Check sheet for the drawn part. Datum: minimum x, y, z corner. Units: mm. Coordinates: 2 decimals unless noted, no trailing zeros. Write each loop counter-clockwise with the first axis right and the second up, starting at its lowest first coordinate (ties: lowest second). Pieces come first, ordered by that corner, then holes. Notation, with made-up numbers: (7.25, -8.5) - (34.25, -8.5) arc R27 ccw to (34.25, 21.5) - close; hole circle Ø10 at (-6, 5.25). An arc over 180 degrees is marked (long way). Write each question's results on one line, items separated by ' | '.
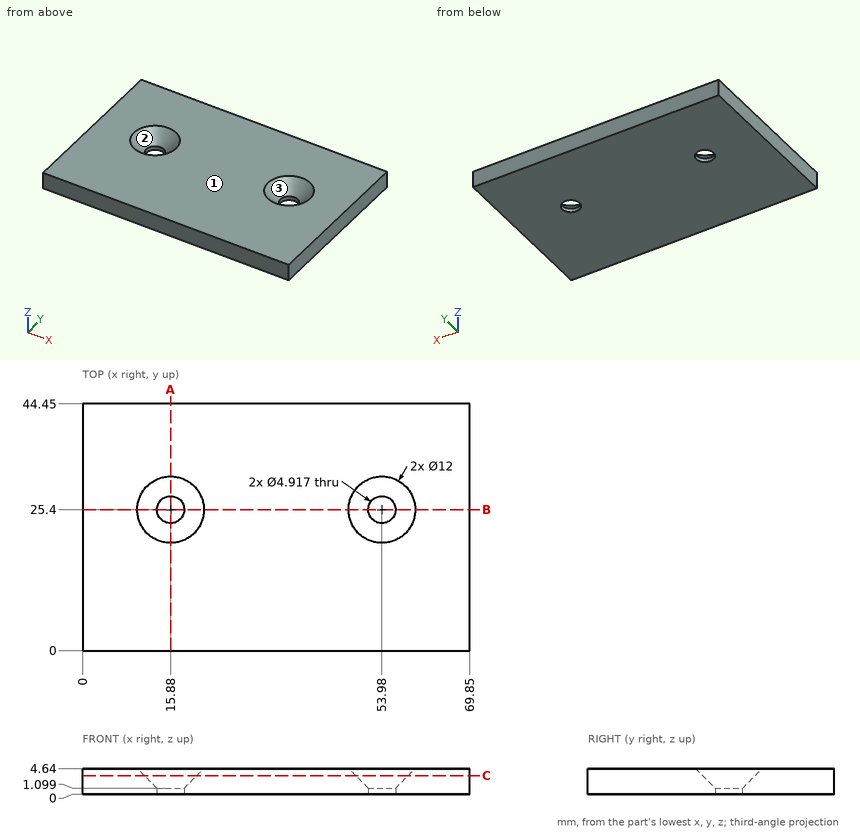
1. Draft check along X on the marked faces 1, 2 and 3. Enter one of: pulls with the +X half, pulls with the -X half, needs draft (parallel to the pull), parting line crosses it, or undercut.
Values follow:
face 1: needs draft | face 2: undercut | face 3: undercut
2. Go/stop test with a flat-tipped pin: pin 1 (2 mm diameter, centred on x = 53.5, y = 13, fed in from -Z). Record where the tip stops, or that it passes through.
Values follow:
pin 1: stops at z = 0
3. Sectioned sample at B-B (y = 25.4). Record the cut outline in (x, z).
Values follow:
outline: (0, 0) - (13.42, 0) - (13.42, 1.1) - (9.88, 4.64) - (0, 4.64) - close; (18.34, 0) - (51.52, 0) - (51.52, 1.1) - (47.98, 4.64) - (21.88, 4.64) - (18.34, 1.1) - close; (56.44, 0) - (69.85, 0) - (69.85, 4.64) - (59.98, 4.64) - (56.44, 1.1) - close
4. Sectioned sample at A-A (x = 15.88). Record the cut outline in (y, z).
Values follow:
outline: (0, 0) - (22.94, 0) - (22.94, 1.1) - (19.4, 4.64) - (0, 4.64) - close; (27.86, 0) - (44.45, 0) - (44.45, 4.64) - (31.4, 4.64) - (27.86, 1.1) - close
5. Material ranges on L1, parallel to X at y = 25.4, z = 0.35; L2, parallel to X at y = 24, z = 3.85; L3, parallel to Y at x = 15.88, z = 0.6, recorded low to high. Write a range as [from, to].
Values follow:
L1: x = [0, 13.42], [18.34, 51.52], [56.44, 69.85] | L2: x = [0, 10.86], [20.9, 48.96], [59, 69.85] | L3: y = [0, 22.94], [27.86, 44.45]
6. Sectioned sample at C-C (z = 3.35). Record the cut outline in (x, y).
Values follow:
outline: (0, 0) - (69.85, 0) - (69.85, 44.45) - (0, 44.45) - close; hole circle Ø9.42 at (15.88, 25.4); hole circle Ø9.42 at (53.98, 25.4)
